CAD build for the part. Positions are in the model's coordinates, mm. Face numbers are marked on the shaded views. A direction names the side the tool comes from. Give positions to 0.01 mm unless a question says otherwise; leave off trailing zeros. Loops run counter-clockwise (first coordinate to the right, second up) from the corner with the lowest first, then second, coordinate; pieces in that order, holes last. Notation, with made-up numbers: M 75,62.25 L 126,62.25 A23 cw 126,80.25 Z; hole C 49,-35.75 d10. An arc over 180 degrees is marked long. Answer as CSV lines item,"result".
```python
from build123d import *

# Parameters (mm, degrees)
SKETCH1_W           = 20
SKETCH1_H           = 20
SKETCH1_R           = 2.5
BOSS_EXTRUDE1_DEPTH = 3
SKETCH2_W           = 20
SKETCH2_H           = 2
BOSS_EXTRUDE2_DEPTH = 25
SKETCH3_R           = 1.5
CUT_EXTRUDE1_DEPTH  = 25


with BuildPart() as part:
    # Sketch1 → Boss-Extrude1 (new body)
    with BuildSketch(Plane(origin=(0, 0, 0), x_dir=(1, 0, 0), z_dir=(0, 1, 0))):
        with Locations((10, 10)):
            Rectangle(SKETCH1_W, SKETCH1_H)
        with Locations(Location((10, 10, 0), (0, 0, 270))):
            Circle(SKETCH1_R, mode=Mode.SUBTRACT)
    extrude(amount=BOSS_EXTRUDE1_DEPTH)

    # Sketch2 → Boss-Extrude2 (add)
    with BuildSketch(Plane(origin=(0, 3, 0), x_dir=(1, 0, 0), z_dir=(0, 1, 0))):
        with Locations((10, 1)):
            Rectangle(SKETCH2_W, SKETCH2_H)
    extrude(amount=BOSS_EXTRUDE2_DEPTH)

    # Sketch3 → Cut-Extrude1 (cut)
    with BuildSketch(Plane.XY):
        with Locations((4, 24)):
            Circle(SKETCH3_R)
        with Locations((16.6, 7)):
            Circle(SKETCH3_R)
        with Locations((3.010167482, 7)):
            Circle(SKETCH3_R)
        with Locations((15.610167482, 24)):
            Circle(SKETCH3_R)
    extrude(amount=-CUT_EXTRUDE1_DEPTH, mode=Mode.SUBTRACT)


solid = part.part
```
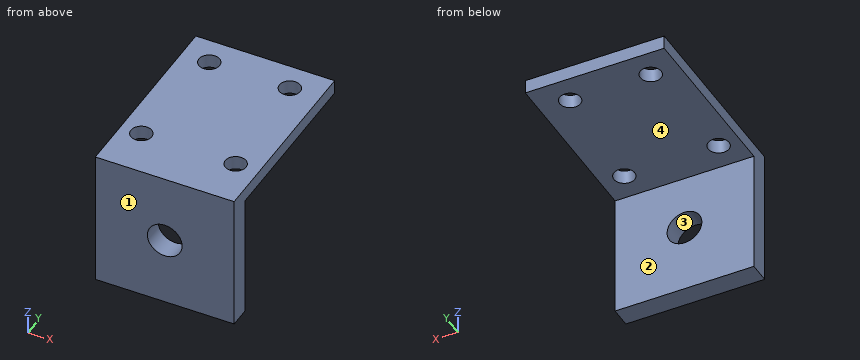
Q1. Mould opens along X. For the marked faces 3 and 4 say: released by +X, released by -X, zero draft, split by the parting line, or undercut.
Solution:
face 3,"undercut"
face 4,"zero draft"
Q2. Wall check: line 1 (Y direction, x = 1.5, z = -15.75); line 2 (Z direction, x = 1.75, y = 22); line 3 (Y direction, x = 16.6, z = -0.95). Give the ranges that are in metal, low to high. Write a range as [from, to].
Solution:
line 1,"y = [0, 3]"
line 2,"z = [-2, 0]"
line 3,"y = [0, 5.5], [8.5, 22.87], [25.13, 28]"
Q3. Pin check, flat tips, straight feed: P1, Ø10, axis at x = 10, y = 13, coming from the -Z side; P2, Ø4, axis at x = 15.5, z = -16.5, coming from the +Y side. Stop position of each tip, or through.
Solution:
P1,"stops at z = -2"
P2,"stops at y = 3"
Q4. Cut at A-A (z = -10). Write the cut outline in (x, y), and give its area (3 significant figures).
Solution:
outline,"M 0,0 L 7.5,0 L 7.5,3 L 0,3 Z; M 12.5,0 L 20,0 L 20,3 L 12.5,3 Z"
area,"45.0 mm²"
Q5. Which spindle directions (+Z, -Z, +X, -X, +Y, -Y) get a long thin tool onto all of the face, cutting with end or side? Do the marked faces 1 and 2. Say none if no direction does.
Solution:
face 1,"+Z, -Z, +X, -X, -Y"
face 2,"-Z, +X, -X, +Y"
Q6. Cut at D-D (x = 16.6). Write the cut outline in (y, z), and give its area (3 significant figures).
Solution:
outline,"M 0,-20 L 3,-20 L 3,-2 L 5.5,-2 L 5.5,0 L 0,0 Z; M 8.5,-2 L 22.87,-2 L 22.87,0 L 8.5,0 Z; M 25.13,-2 L 28,-2 L 28,0 L 25.13,0 Z"
area,"99.5 mm²"
Q7. Cut at C-C (x = 10). Write the cut outline in (y, z).
Solution:
outline,"M 0,-20 L 3,-20 L 3,-12.5 L 0,-12.5 Z; M 0,-7.5 L 3,-7.5 L 3,-2 L 28,-2 L 28,0 L 0,0 Z"
Q8. Cut at B-B (y = 24). Write the cut outline in (x, z), and give its area (3 significant figures).
Solution:
outline,"M 0,-2 L 2.5,-2 L 2.5,0 L 0,0 Z; M 5.5,-2 L 14.11,-2 L 14.11,0 L 5.5,0 Z; M 17.11,-2 L 20,-2 L 20,0 L 17.11,0 Z"
area,"28.0 mm²"
